Source: three-view drawing plus pictorial views. Frame: mm from the lowest corner of the part. A direction names the side the tool comes from. Give positions to 0.01 mm unless a question says otherwise; leave off trailing zeros. Loops run counter-clockwise (first coordinate to the right, second up) from the corner with the lowest first, then second, coordinate; pieces in that order, holes last. Notation, with made-up numbers: (51.25, -27.75) - (93.25, -27.75) arc R22 ccw to (93.25, 6.25) - close; hole circle Ø10 at (53.5, -30). An arc over 180 degrees is marked (long way). Answer as a JSON object with one key per item and string values. Group by question number.
(1) Access query for the marked faces 1 and 2. Directions: +Z, -Z, +X, -X, +Y, -Y. A direction counts if a zero-diameter tool reaches every point of the face in a straight line with its end or side. Return the directions, or none.
(2) Pin query (flat end, axial travel): P1, Ø2.5, axis at x = 96.5, z = 27, coming from the +Y side; P2, Ø2.5, axis at y = 55, z = 25, coming from the -X side; P3, Ø10, axis at x = 38, y = 50.5, coming from the +Z side; P4, Ø3, axis at x = 30.5, y = 10.5, coming from the -Z side. Return the tip coordinate at first contact, or that it passes through.
(3) Section query A-A (z = 15.75). Return loops of the section in (x, y).
(4) Section query C-C (y = 9.5). Return loops of the section in (x, z).
(5) Section query D-D (x = 91). Return loops of the section in (y, z).
(6) Mould query, pull axis Y, two halves, no side actions, for the marked faces 3, 4 and 5. Classes: +Y half, -Y half, draft (parallel to the pull), parting line (faces both ways), or undercut.
(7) Section query B-B (x = 26). Return loops of the section in (y, z).
(8) Material intervals for L1, parallel to Y at x = 7.5, z = 25; L2, parallel to Y at x = 81, z = 24.25; L3, parallel to X at y = 14, z = 8.5, sorted ascending.
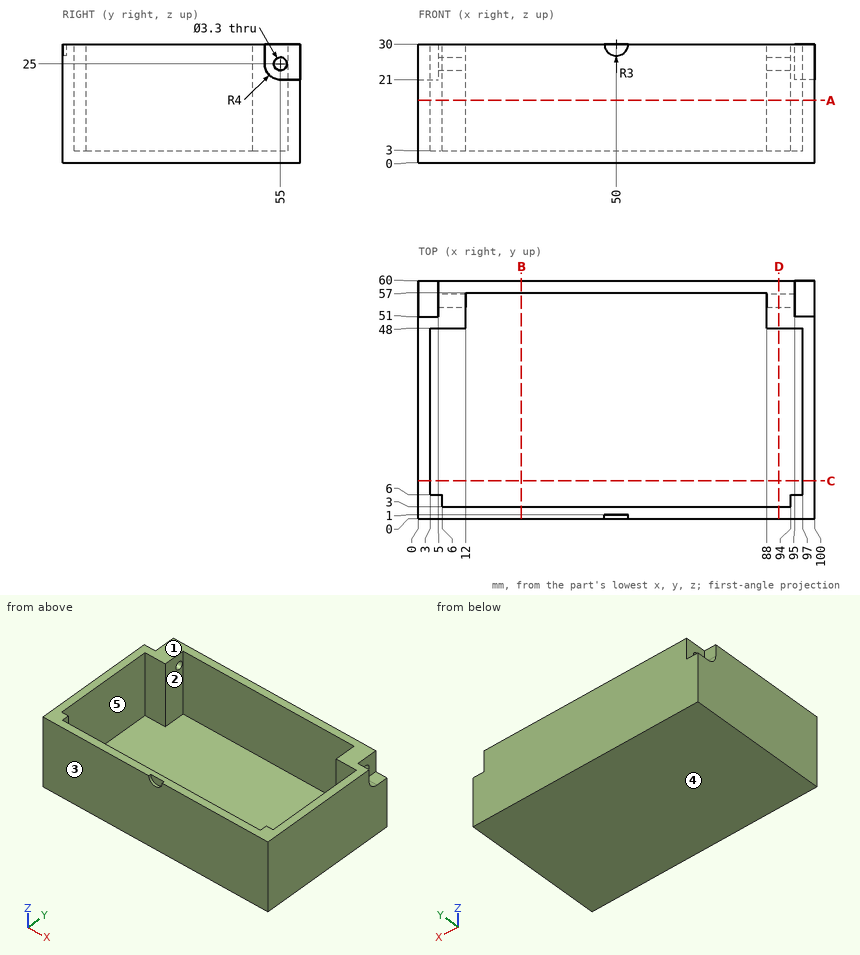
Recorded:
{
 "1": {"face 1": "+Z, +X, -X, +Y, -Y", "face 2": "+Z"},
 "2": {"P1": "stops at y = 51", "P2": "passes through", "P3": "stops at z = 3", "P4": "stops at z = 0"},
 "3": {"outline": "(0, 0) - (100, 0) - (100, 60) - (0, 60) - close; hole (3, 6) - (6, 6) - (6, 3) - (94, 3) - (94, 6) - (97, 6) - (97, 48) - (88, 48) - (88, 57) - (12, 57) - (12, 48) - (3, 48) - close"},
 "4": {"outline": "(0, 0) - (100, 0) - (100, 30) - (97, 30) - (97, 3) - (3, 3) - (3, 30) - (0, 30) - close"},
 "5": {"outline": "(0, 0) - (60, 0) - (60, 30) - (48, 30) - (48, 3) - (3, 3) - (3, 30) - (0, 30) - close; hole circle Ø3.3 at (55, 25)"},
 "6": {"face 3": "-Y half", "face 4": "draft", "face 5": "undercut"},
 "7": {"outline": "(0, 0) - (60, 0) - (60, 30) - (57, 30) - (57, 3) - (3, 3) - (3, 30) - (0, 30) - close"},
 "8": {"L1": "y = 0 to 3, 48 to 53.35, 56.65 to 60", "L2": "y = 0 to 3, 57 to 60", "L3": "x = 0 to 3, 97 to 100"}
}
